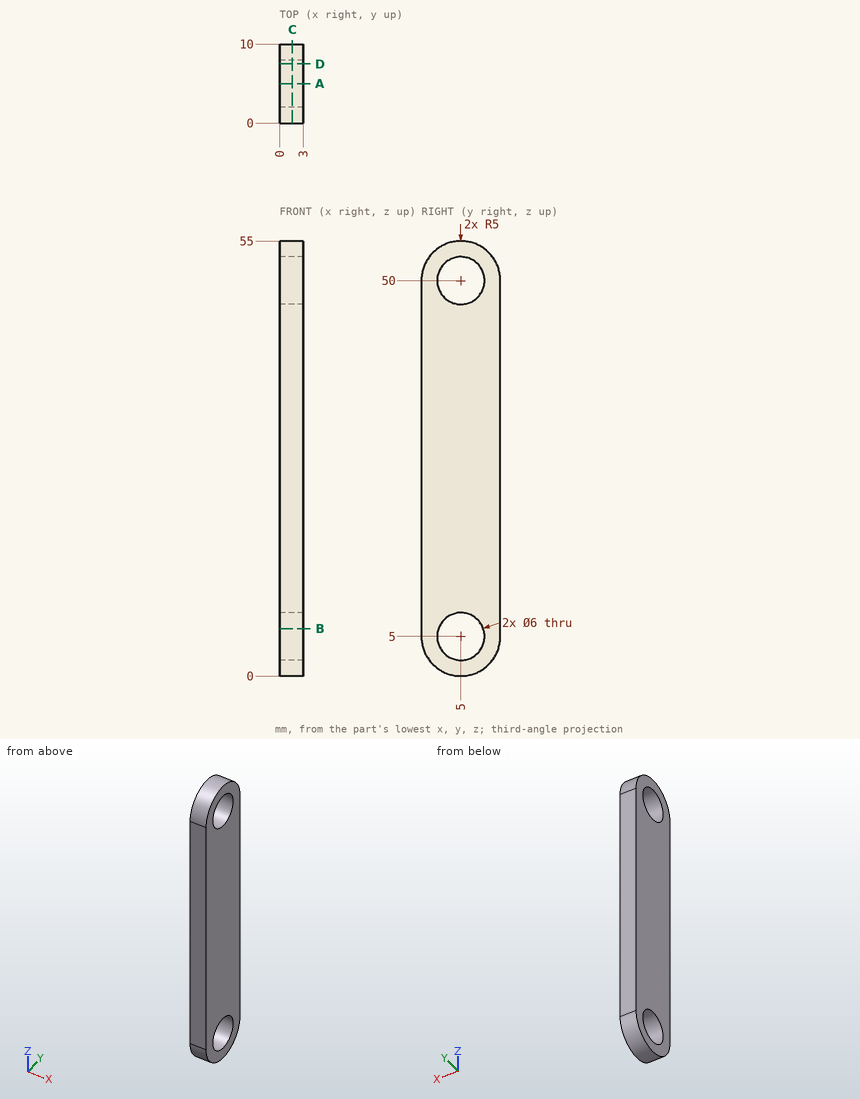
Study the drawing (mm; zero at the part's minimum x, y, z) and answer. Give positions to 0.01 mm unless a question says otherwise; leave off trailing zeros. Write each loop counter-clockwise with the first axis right and the second up, starting at its lowest first coordinate (ties: lowest second). Pieces come first, ordered by that corner, then holes. Notation, with made-up numbers: (-29.5, -34.5) -> (12.5, -34.5) arc R30 cw to (12.5, 1.5) -> close; hole circle Ø2 at (60.25, -36.75). An arc over 180 degrees is marked (long way). Answer as a JSON object with one key per item and string values. Group by question number.
1) Find section C-C (x = 1.6). Write down the section's boundary in (y, z), and give its area (3 significant figures).
2) Each of these flat-tipped pins is pushed along its axis until it touches: P1, Ø1, axis at x = 1.5, y = 6.5, coming from the +Z side; P2, Ø4, axis at y = 2.5, z = 43.5, coming from the -X side. Where does it stop, or does it pass through?
3) Consider L1, parallel to Z at x = 1.65, y = 5; L2, parallel to Z at x = 1.85, y = 2.5; L3, parallel to Y at x = 1.85, z = 52.5. Determine where each line is inside the solid, lowest interval first. Write a range as from..to.
4) Find section B-B (z = 6). Write down the section's boundary in (x, y).
5) Find section D-D (y = 7.5). Write down the section's boundary in (x, z).
6) Find section A-A (y = 5). Write down the section's boundary in (x, z), and give its area (3 significant figures).
Values follow:
{
 "1": {"outline": "(0, 5) arc R5 ccw to (10, 5) -> (10, 50) arc R5 ccw to (0, 50) -> close; hole circle Ø6 at (5, 5); hole circle Ø6 at (5, 50)", "area": "472 mm2"},
 "2": {"P1": "stops at z = 54.9", "P2": "stops at x = 0"},
 "3": {"L1": "z = 0..2, 8..47, 53..55", "L2": "z = 0.67..3.34, 6.66..48.34, 51.66..54.33", "L3": "y = 0.67..3.34, 6.66..9.33"},
 "4": {"outline": "(0, 0) -> (3, 0) -> (3, 2.17) -> (0, 2.17) -> close; (0, 7.83) -> (3, 7.83) -> (3, 10) -> (0, 10) -> close"},
 "5": {"outline": "(0, 0.67) -> (3, 0.67) -> (3, 3.34) -> (0, 3.34) -> close; (0, 6.66) -> (3, 6.66) -> (3, 48.34) -> (0, 48.34) -> close; (0, 51.66) -> (3, 51.66) -> (3, 54.33) -> (0, 54.33) -> close"},
 "6": {"outline": "(0, 0) -> (3, 0) -> (3, 2) -> (0, 2) -> close; (0, 8) -> (3, 8) -> (3, 47) -> (0, 47) -> close; (0, 53) -> (3, 53) -> (3, 55) -> (0, 55) -> close", "area": "129 mm2"}
}
